Could you check a few things on this model? Use its own coordinates, in mm. Face numbers are marked on the shaded views. A direction names the side the tool comes from. Round coordinates to 2 decimals unless told otherwise and drop trailing zeros. Write each loop counter-clockwise with the first axis right and the second up, starting at its lowest first coordinate (ties: lowest second). Pieces come first, ordered by that corner, then holes. Notation, with made-up numbers: (79.25, -15) - (110.25, -15) arc R32 ccw to (110.25, 17) - close; hole circle Ø3 at (2.5, 83.5). An arc over 180 degrees is marked (long way). Write each question's results on one line, items separated by ' | '. Start each with the question number.
(1) Imagine slicing it at D-D on y = 5. State how many separate pieces and enclosed holes the cut face has, then the cut area to 3 significant figures.
(2) Imagine slicing it at A-A on x = 0. Write out the boundary of the cut face in (y, z) (3 decimals), then the cut area to 4 significant figures.
(3) On a 3-axis mill with a long thin cutter (end or side, diameter ignored), from which of +Z, -Z, +X, -X, +Y, -Y can I reach the whole of each face in a straight line? I mean the marked faces 4 and 5. Say none if no direction works.
(4) Please list where these lines run through material, in increasing order: line 1 (Z direction, x = 0, y = -7) (3 decimals); line 2 (Z direction, x = -19.5, y = -13); line 3 (X direction, y = -6, z = 2) (3 decimals). Write a range as [from, to].
(5) Imagine slicing it at C-C on z = 16. Write out the boundary of the cut face in (x, y).
(6) Thinking about a two-plate mould opening in Y: for the marked faces 1, 2 and 3, which applies, +Y half, -Y half, draft (parallel to the pull), parting line (faces both ways), or undercut?
(7) For P1, Ø0.8, axis at x = 11, z = 10.5, coming from the +Y side; P2, Ø8, axis at x = 7, z = -11.5, coming from the -Y side; P3, Ø1.2, axis at x = -18, y = -3.5, coming from the -Z side; P4, Ø1.5, axis at x = 12, y = -2.5, coming from the -Z side, each with a flat end and sliding along its axis, tell me the tip position at first contact or that it passes through.
(8) Imagine slicing it at B-B on z = 0. Write out the boundary of the cut face in (x, y) (3 decimals), then the cut area to 3 significant figures.
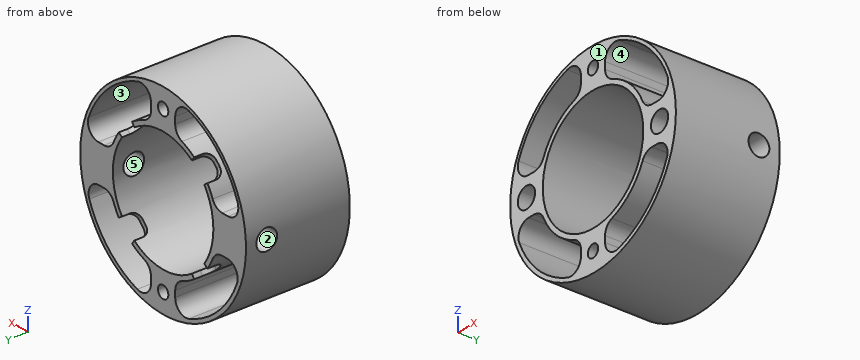
```python
from build123d import *

# Parameters (mm, degrees)
SKETCH3_R                = 24
SKETCH3_R_2              = 14.55
BOSS_EXTRUDE1_DEPTH      = 10
BOSS_EXTRUDE1_DEPTH_BACK = 15
CUT_EXTRUDE2_START       = 50
SKETCH4_R                = 2.5
CUT_EXTRUDE2_DEPTH       = 100
SKETCH5_R                = 1.5
CUT_EXTRUDE3_DEPTH       = 100
CUT_EXTRUDE6_DEPTH       = 26
CUT_EXTRUDE7_DEPTH       = 26
CUT_EXTRUDE8_DEPTH       = 26
CUT_EXTRUDE9_DEPTH       = 26
FILLET5_R                = 3
CUT_EXTRUDE12_DEPTH      = 4
FILLET10_R               = 2
SKETCH20_R               = 2.5
CUT_EXTRUDE13_DEPTH      = 15


with BuildPart() as part:
    # Sketch3 → Boss-Extrude1 (new body, two sides)
    with BuildSketch(Plane(origin=(0, 0, 0), x_dir=(1, 0, 0), z_dir=(0, 1, 0))) as boss_extrude1_sk:
        Circle(SKETCH3_R)
        Circle(SKETCH3_R_2, mode=Mode.SUBTRACT)
    extrude(amount=BOSS_EXTRUDE1_DEPTH)
    extrude(boss_extrude1_sk.sketch, amount=-BOSS_EXTRUDE1_DEPTH_BACK)

    # Sketch4 → Cut-Extrude2 (cut)
    with BuildSketch(Plane(origin=(0, 0, 0), x_dir=(0, 0, -1), z_dir=(1, 0, 0)).offset(CUT_EXTRUDE2_START)):
        with Locations((0, 5)):
            Circle(SKETCH4_R)
    extrude(amount=-CUT_EXTRUDE2_DEPTH, mode=Mode.SUBTRACT)

    # Sketch5 → Cut-Extrude3 (cut)
    with BuildSketch(Plane(origin=(0, 10, 0), x_dir=(1, 0, 0), z_dir=(0, 1, 0))):
        with Locations((0, 19.275)):
            Circle(SKETCH5_R)
        with Locations((0, -19.275)):
            Circle(SKETCH5_R)
    extrude(amount=-CUT_EXTRUDE3_DEPTH, mode=Mode.SUBTRACT)

    # Sketch7 → Cut-Extrude6 (cut)
    with BuildSketch(Plane(origin=(0, 10, 0), x_dir=(1, 0, 0), z_dir=(0, 1, 0))):
        with BuildLine():
            Line((3.5, 15.275), (3.5, 22.775))
            ThreePointArc((3.5, 22.775), (15.930450829, 16.648464235), (22.598686356, 4.5))
            Line((22.598686356, 4.5), (15.010850242, 4.5))
            ThreePointArc((15.010850242, 4.5), (10.709250694, 11.440610761), (3.5, 15.275))
        make_face()
    extrude(amount=-CUT_EXTRUDE6_DEPTH, mode=Mode.SUBTRACT)

    # Sketch9 → Cut-Extrude7 (cut)
    with BuildSketch(Plane(origin=(0, 10, 0), x_dir=(1, 0, 0), z_dir=(0, 1, 0))):
        with BuildLine():
            Line((15.010850242, -4.5), (22.775, -4.5))
            ThreePointArc((22.775, -4.5), (16.052855024, -16.770702746), (3.5, -22.94995915))
            Line((3.5, -22.94995915), (3.5, -15.275))
            ThreePointArc((3.5, -15.275), (10.709250694, -11.440610761), (15.010850242, -4.5))
        make_face()
    extrude(amount=-CUT_EXTRUDE7_DEPTH, mode=Mode.SUBTRACT)

    # Sketch10 → Cut-Extrude8 (cut)
    with BuildSketch(Plane(origin=(0, 10, 0), x_dir=(1, 0, 0), z_dir=(0, 1, 0))):
        with BuildLine():
            Line((-3.5, 15.275), (-3.5, 22.775))
            ThreePointArc((-3.5, 22.775), (-15.930450829, 16.648464235), (-22.598686356, 4.5))
            Line((-22.598686356, 4.5), (-15.010850242, 4.5))
            ThreePointArc((-15.010850242, 4.5), (-10.709250694, 11.440610761), (-3.5, 15.275))
        make_face()
    extrude(amount=-CUT_EXTRUDE8_DEPTH, mode=Mode.SUBTRACT)

    # Sketch11 → Cut-Extrude9 (cut)
    with BuildSketch(Plane(origin=(0, 10, 0), x_dir=(1, 0, 0), z_dir=(0, 1, 0))):
        with BuildLine():
            Line((-15.010850242, -4.5), (-22.775, -4.5))
            ThreePointArc((-22.775, -4.5), (-16.052855024, -16.770702746), (-3.5, -22.94995915))
            Line((-3.5, -22.94995915), (-3.5, -15.275))
            ThreePointArc((-3.5, -15.275), (-10.709250694, -11.440610761), (-15.010850242, -4.5))
        make_face()
    extrude(amount=-CUT_EXTRUDE9_DEPTH, mode=Mode.SUBTRACT)

    # Fillet5
    fillet5_edges = [part.edges().sort_by_distance(p)[0] for p in [
        (-3.5, -2.5, 22.94995915),
        (-22.775, -2.5, 4.5),
        (-15.010850242, -2.5, 4.5),
        (-3.5, -2.5, 15.275),
        (3.5, -2.5, -22.775),
        (22.598686356, -2.5, -4.5),
        (15.010850242, -2.5, -4.5),
        (3.5, -2.5, -15.275),
        (3.5, -2.5, 15.275),
        (15.010850242, -2.5, 4.5),
        (22.775, -2.5, 4.5),
        (3.5, -2.5, 22.94995915),
        (-3.5, -2.5, -15.275),
        (-15.010850242, -2.5, -4.5),
        (-22.598686356, -2.5, -4.5),
        (-3.5, -2.5, -22.775),
    ]]
    fillet(fillet5_edges, radius=FILLET5_R)

    # Sketch19 → Cut-Extrude12 (cut)
    with BuildSketch(Plane(origin=(0, 10, 0), x_dir=(1, 0, 0), z_dir=(0, 1, 0))):
        with BuildLine():
            Line((-12.836811042, 8.988431858), (-11.918662244, 8.345537149))
            ThreePointArc((-11.918662244, 8.345537149), (-10.288403666, 10.288403666), (-8.345537149, 11.918662244))
            Line((-8.345537149, 11.918662244), (-8.988431858, 12.836811042))
            ThreePointArc((-8.988431858, 12.836811042), (-11.080966226, 11.080966226), (-12.836811042, 8.988431858))
        make_face()
        with BuildLine():
            Line((8.988431858, 12.836811042), (8.345537149, 11.918662244))
            ThreePointArc((8.345537149, 11.918662244), (10.288403666, 10.288403666), (11.918662244, 8.345537149))
            Line((11.918662244, 8.345537149), (12.836811042, 8.988431858))
            ThreePointArc((12.836811042, 8.988431858), (11.080966226, 11.080966226), (8.988431858, 12.836811042))
        make_face()
        with BuildLine():
            ThreePointArc((11.918662244, -8.345537149), (10.288403666, -10.288403666), (8.345537149, -11.918662244))
            Line((8.345537149, -11.918662244), (8.988431858, -12.836811042))
            ThreePointArc((8.988431858, -12.836811042), (11.080966226, -11.080966226), (12.836811042, -8.988431858))
            Line((12.836811042, -8.988431858), (11.918662244, -8.345537149))
        make_face()
        with BuildLine():
            Line((-8.988431858, -12.836811042), (-8.345537149, -11.918662244))
            ThreePointArc((-8.345537149, -11.918662244), (-10.288403666, -10.288403666), (-11.918662244, -8.345537149))
            Line((-11.918662244, -8.345537149), (-12.836811042, -8.988431858))
            ThreePointArc((-12.836811042, -8.988431858), (-11.080966226, -11.080966226), (-8.988431858, -12.836811042))
        make_face()
    extrude(amount=-CUT_EXTRUDE12_DEPTH, mode=Mode.SUBTRACT)

    # Fillet10
    fillet10_edges = [part.edges().sort_by_distance(p)[0] for p in [
        (-12.377736643, 6, 8.666984504),
        (-8.666984504, 6, 12.377736643),
        (8.666984504, 6, 12.377736643),
        (12.377736643, 6, 8.666984504),
        (12.377736643, 6, -8.666984504),
        (8.666984504, 6, -12.377736643),
        (-8.666984504, 6, -12.377736643),
        (-12.377736643, 6, -8.666984504),
    ]]
    fillet(fillet10_edges, radius=FILLET10_R)

    # Sketch20 → Cut-Extrude13 (cut)
    with BuildSketch(Plane.XZ.offset(15)):
        with Locations((-19.275, 0)):
            Circle(SKETCH20_R)
        with Locations((19.275, 0)):
            Circle(SKETCH20_R)
    extrude(amount=-CUT_EXTRUDE13_DEPTH, mode=Mode.SUBTRACT)


solid = part.part
```
Response:
1) separate pieces: 2 | enclosed holes: 6 | area: 403 mm²
2) outline: (-15, -24) - (10, -24) - (10, -20.775) - (-15, -20.775) - close; (-15, -17.775) - (10, -17.775) - (10, -14.55) - (-15, -14.55) - close; (-15, 14.55) - (10, 14.55) - (10, 17.775) - (-15, 17.775) - close; (-15, 20.775) - (10, 20.775) - (10, 24) - (-15, 24) - close | area: 322.5 mm²
3) face 4: +Y, -Y | face 5: +X, -X
4) line 1: [-24, -20.775], [-17.775, -14.55], [14.55, 17.775], [20.775, 24] | line 2: [-13.99, -12.28], [-4.64, -2.49], [2.49, 4.59], [12.6, 13.99] | line 3: [-23.917, -20.775], [-17.775, -14.412], [14.412, 17.775], [20.775, 23.917]
5) outline: (-17.89, -15) - (-16.82, -15) - (-16.82, 10) - (-17.89, 10) - close; (-3.9, -15) - (3.9, -15) - (3.9, 10) - (-3.9, 10) - close; (16.82, -15) - (17.89, -15) - (17.89, 10) - (16.82, 10) - close
6) face 1: -Y half | face 2: undercut | face 3: draft
7) P1: y = 6 | P2: y = -15 | P3: z = -16.53 | P4: z = -21.2
8) outline: (-24, -15) - (-21.775, -15) - (-21.775, 0) - (-16.775, 0) - (-16.775, -15) - (-14.55, -15) - (-14.55, 2.5) - (-24, 2.5) - close; (-24, 7.5) - (-14.55, 7.5) - (-14.55, 10) - (-24, 10) - close; (14.55, -15) - (16.775, -15) - (16.775, 0) - (21.775, 0) - (21.775, -15) - (24, -15) - (24, 2.5) - (14.55, 2.5) - close; (14.55, 7.5) - (24, 7.5) - (24, 10) - (14.55, 10) - close | area: 228 mm²
